```python
from build123d import *

# Parameters (mm, degrees)
F0_W      = 130
F0_H      = 130
F1_DEPTH  = 60
F2_W      = 110
F2_H      = 110
F3_DEPTH  = 50
F4_W      = 89
F4_H      = 40
F5_DEPTH  = 4
F6_R      = 7
F7_W      = 10
F7_H      = 4
F8_DEPTH  = 4
F9_W      = 10
F9_H      = 4
F10_DEPTH = 4
F11_W     = 10
F11_H     = 10
F12_DEPTH = 4
F15_DEPTH = 5
F17_R     = 3.7840755507
F18_DEPTH = 10


with BuildPart() as f1:
    # F0 (on Top) → F1 (new body)
    with BuildSketch(Plane.XY):
        Rectangle(F0_W, F0_H)
    extrude(amount=F1_DEPTH)

    # F2 (on Top) → F3 (cut)
    with BuildSketch(Plane.XY):
        Rectangle(F2_W, F2_H)
    extrude(amount=F3_DEPTH, mode=Mode.SUBTRACT)

    # F4 (on face) → F5 (cut)
    with BuildSketch(Plane.XY.offset(60)):
        with Locations((20.5, 0)):
            Rectangle(F4_W, F4_H)
    extrude(amount=-F5_DEPTH, mode=Mode.SUBTRACT)

    # F6
    f6_edges = [f1.edges().sort_by_distance(p)[0] for p in [
        (55, -55, 25),
        (55, 55, 25),
        (-55, 55, 25),
        (-55, -55, 25),
    ]]
    fillet(f6_edges, radius=F6_R)

    # F7 (on face) → F8 (cut)
    with BuildSketch(Plane.XY):
        with Locations((-60, -39.7807884514)):
            Rectangle(F7_W, F7_H)
    extrude(amount=F8_DEPTH, mode=Mode.SUBTRACT)

    # F9 (on face) → F10 (cut)
    with BuildSketch(Plane.XY):
        with Locations((-60, -47.1367839277)):
            Rectangle(F9_W, F9_H)
    extrude(amount=F10_DEPTH, mode=Mode.SUBTRACT)

    # F11 (on face) → F12 (cut)
    with BuildSketch(Plane.XY):
        with Locations((-60, 45)):
            Rectangle(F11_W, F11_H)
    extrude(amount=F12_DEPTH, mode=Mode.SUBTRACT)

    # F14 (on offset) → F15 (cut)
    with BuildSketch(Plane(origin=(-55, 0, 0), x_dir=(0, -1, 0), z_dir=(-1, 0, 0))):
        with BuildLine():
            ThreePointArc((-2.8704081755, 30), (-0.3704081755, 25), (2.1295918245, 30))
            Line((2.1295918245, 30), (-2.8704081755, 30))
        make_face()
    extrude(amount=F15_DEPTH, mode=Mode.SUBTRACT)

    # F17 (on offset) → F18 (cut)
    with BuildSketch(Plane(origin=(-60, 0, 0), x_dir=(0, -1, 0), z_dir=(-1, 0, 0))):
        with Locations((-0.3525029916, 28.0889305786)):
            Circle(F17_R)
    extrude(amount=F18_DEPTH, mode=Mode.SUBTRACT)


solid = f1.part
```
Source: CAD feature listing. Evaluate the final solid. Frame: model axes, mm. A direction names the side the tool comes from. Coordinates: 2 decimals unless noted, no trailing zeros. Write each loop counter-clockwise with the first axis right and the second up, starting at its lowest first coordinate (ties: lowest second). Pieces come first, ordered by that corner, then holes. Notation, with made-up numbers: (-28.5, -6) - (10.5, -6) arc R33 cw to (10.5, 25) - close; hole circle Ø2 at (34, 53.5). An arc over 180 degrees is marked (long way). Answer as a JSON object with one key per item and string values.
Q1. Section query A-A, the plane y = 18. Output: boundary loops of the cut face in (x, z).
Ans:
{"outline": "(-65, 0) - (-55, 0) - (-55, 50) - (55, 50) - (55, 0) - (65, 0) - (65, 56) - (-24, 56) - (-24, 60) - (-65, 60) - close"}
Q2. Material intervals for line 1 (X direction, y = -15, z = 25.5); line 2 (Z direction, x = -35.5, y = -44), sorted ascending. Write a range as [from, to].
Ans:
{"line 1": "x = [-65, -55], [55, 65]", "line 2": "z = [50, 60]"}
Q3. Draft query along Y for faces 1 (the cylindrical face through (-62.46, 0.85, 31.84)), 2 (the flat face through (57, 0, 0)), 3 (the cylindrical face through (-52.9, -53, 25.4)). Return one class per face: released by +Y, released by -Y, zero draft, split by the parting line, or undercut.
Ans:
{"face 1": "undercut", "face 2": "zero draft", "face 3": "undercut"}
Q4. Section query D-D, the plane y = -25. Output: boundary loops of the cut face in (x, z), plus the area to 3 significant figures.
Ans:
{"outline": "(-65, 0) - (-55, 0) - (-55, 50) - (55, 50) - (55, 0) - (65, 0) - (65, 60) - (-65, 60) - close", "area": "2,300 mm2"}
Q5. Set-up query: faces 4 (the flat face through (-60, 0.1, 30.3)), 5 (the cylindrical face through (-52.9, 53, 25.4)), 6 (the flat face through (-60, -49.137, 2)). Return all of +Z, -Z, +X, -X, +Y, -Y with unobstructed straight access to the full face (end or side cutting, diameter ignored); none if empty.
Ans:
{"face 4": "-X", "face 5": "-Z", "face 6": "-Z, -X"}
Q6. Section query B-B, the plane z = 47. Output: boundary loops of the cut face in (x, y), plus the area to 3 significant figures.
Ans:
{"outline": "(-65, -65) - (65, -65) - (65, 65) - (-65, 65) - close; hole (-55, -48) arc R7 ccw to (-48, -55) - (48, -55) arc R7 ccw to (55, -48) - (55, 48) arc R7 ccw to (48, 55) - (-48, 55) arc R7 ccw to (-55, 48) - close", "area": "4,840 mm2"}
Q7. Section query C-C, the plane x = 31. Output: boundary loops of the cut face in (y, z), plus the area to 3 significant figures.
Ans:
{"outline": "(-65, 0) - (-55, 0) - (-55, 50) - (55, 50) - (55, 0) - (65, 0) - (65, 60) - (20, 60) - (20, 56) - (-20, 56) - (-20, 60) - (-65, 60) - close", "area": "2,140 mm2"}
Q8. First-contact query: pin 1 Ø12 at (x, y) = (38, -6.5) entering from +Z; pin 2 Ø3 at (x, y) = (-61, -40) entering from -Z; pin 3 Ø2.5 at (y, z) = (2, 28) entering from -X. Flat tips, straight axial feed; report the tip coordinate or a pass-through.
Ans:
{"pin 1": "stops at z = 56", "pin 2": "stops at z = 4", "pin 3": "stops at x = 55"}
